Could you check a few things on this model? Use its own coordinates, in mm. Face numbers are marked on the shaded views. Give positions to 0.01 mm unless a question says otherwise; leave off trailing zeros. Loops run counter-clockwise (first coordinate to the right, second up) from the corner with the lowest first, then second, coordinate; pieces in that order, holes last. Notation, with made-up numbers: (23.25, 25.25) -> (71.25, 25.25) arc R22 ccw to (71.25, 50.25) -> close; hole circle Ø3 at (63.25, 20). An arc over 180 degrees is marked (long way). Write each question's results on one line, items separated by ' | '. Start each with the question number.
Q1. If we section it at C-C, the plane y = 322.5: List the corners of the cut face in (x, z) for me, plus the area to 3 significant figures.
Q2. If we section it at B-B, the plane x = 200: List the corners of the cut face in (y, z) for me, plus the area to 3 significant figures.
Q3. If we section it at D-D, the plane y = 122: List the corners of the cut face in (x, z) for me, plus the area to 3 significant figures.
Q4. Will these pins go through, and if not, where does the flat tip stop? P1, Ø12, axis at y = 168, z = 24.5, coming from the -X side; P2, Ø8, axis at x = 69.5, y = 121.5, coming from the +Z side; P3, Ø6.5, axis at y = 346.5, z = 16.5, coming from the -X side; P4, Ø4, axis at y = 351.47, z = 38.1, coming from the +X side.
Q5. If I drill on line 1 along Z through (x, y) = (76.5, 195.5); line 2 along X through (y, z) = (114, 5.5); line 3 along X through (y, z) = (356, 54), over which ranges is the centre line in solid material (lowest first)?
Q6. We'd pull the mould along Y, two halves only. Please class the marked faces 1, 2 and 3: released by +Y, released by -Y, zero draft, split by the parting line, or undercut.
Q7. If we section it at A-A, the plane z = 20: List the corners of the cut face in (x, y) for me (3 decimals), plus the area to 3 significant figures.
from build123d import *

# Parameters (mm, degrees)
F1_DEPTH = 12.7
F2_W     = 25.4
F2_H     = 50.8
F3_DEPTH = 63.5
F4_SIZE  = 20.32
F5_SIZE  = 17.78
F7_DEPTH = 254
F9_DEPTH = 254


with BuildPart() as f1:
    # F0 (on Top) → F1 (new body)
    with BuildSketch(Plane.XY):
        Polygon((50.8, 190.5), (114.3, 190.5), (114.3, 381), (0, 381), (0, 292.1), (50.8, 292.1), align=None)
        Polygon((114.3, 381), (114.3, 190.5), (177.8, 190.5), (177.8, 292.1), (228.6, 292.1), (228.6, 381), align=None)
        Polygon((0, 88.9), (0, 0), (114.3, 0), (114.3, 190.5), (50.8, 190.5), (50.8, 88.9), align=None)
        Polygon((114.3, 190.5), (114.3, 0), (228.6, 0), (228.6, 88.9), (177.8, 88.9), (177.8, 190.5), align=None)
    extrude(amount=F1_DEPTH)

    # F2 (on Top) → F3 (join)
    with BuildSketch(Plane.XY):
        with Locations((139.7, 339.725)):
            Rectangle(F2_W, F2_H)
        with Locations((88.9, 339.725)):
            Rectangle(F2_W, F2_H)
        with Locations((139.7, 41.275)):
            Rectangle(F2_W, F2_H)
        with Locations((88.9, 41.275)):
            Rectangle(F2_W, F2_H)
    extrude(amount=F3_DEPTH)

    # F4
    f4_edges = [f1.edges().sort_by_distance(p)[0] for p in [
        (101.6, 41.275, 63.5),
        (127, 41.275, 63.5),
        (127, 339.725, 63.5),
        (101.6, 339.725, 63.5),
    ]]
    chamfer(f4_edges, length=F4_SIZE)

    # F5
    f5_edges = [f1.edges().sort_by_distance(p)[0] for p in [
        (127, 339.725, 43.18),
        (101.6, 339.725, 43.18),
        (127, 41.275, 43.18),
        (101.6, 41.275, 43.18),
    ]]
    chamfer(f5_edges, length=F5_SIZE)

    # F6 (on face) → F7 (cut)
    with BuildSketch(Plane(origin=(76.2, 0, 0), x_dir=(0, -1, 0), z_dir=(-1, 0, 0))):
        with BuildLine():
            ThreePointArc((-40.005, 48.1965), (-40.3769743879, 49.0945256121), (-41.275, 49.4665))
            Line((-41.275, 49.4665), (-41.275, 46.9265))
            ThreePointArc((-41.275, 46.9265), (-40.3769743879, 47.2984743879), (-40.005, 48.1965))
        make_face()
        with BuildLine():
            Line((-41.275, 46.9265), (-41.275, 49.4665))
            ThreePointArc((-41.275, 49.4665), (-42.545, 48.1965), (-41.275, 46.9265))
        make_face()
        with BuildLine():
            ThreePointArc((-51.7525, 38.1), (-53.0225, 39.37), (-54.2925, 38.1))
            Line((-54.2925, 38.1), (-51.7525, 38.1))
        make_face()
        with BuildLine():
            Line((-51.7525, 38.1), (-54.2925, 38.1))
            ThreePointArc((-54.2925, 38.1), (-53.0225, 36.83), (-51.7525, 38.1))
        make_face()
        with BuildLine():
            ThreePointArc((-39.243, 38.1), (-39.8381590206, 39.5368409794), (-41.275, 40.132))
            Line((-41.275, 40.132), (-41.275, 38.1))
            Line((-41.275, 38.1), (-39.243, 38.1))
        make_face()
        with BuildLine():
            Line((-41.275, 38.1), (-41.275, 40.132))
            ThreePointArc((-41.275, 40.132), (-42.7118409794, 39.5368409794), (-43.307, 38.1))
            Line((-43.307, 38.1), (-41.275, 38.1))
        make_face()
        with BuildLine():
            Line((-41.275, 38.1), (-43.307, 38.1))
            ThreePointArc((-43.307, 38.1), (-42.7118409794, 36.6631590206), (-41.275, 36.068))
            Line((-41.275, 36.068), (-41.275, 38.1))
        make_face()
        with BuildLine():
            ThreePointArc((-41.275, 29.2735), (-42.545, 28.0035), (-41.275, 26.7335))
            Line((-41.275, 26.7335), (-41.275, 29.2735))
        make_face()
        with BuildLine():
            Line((-41.275, 29.2735), (-41.275, 26.7335))
            ThreePointArc((-41.275, 26.7335), (-40.3769743879, 27.1054743879), (-40.005, 28.0035))
            ThreePointArc((-40.005, 28.0035), (-40.3769743879, 28.9015256121), (-41.275, 29.2735))
        make_face()
        with BuildLine():
            Line((-30.7975, 38.1), (-28.2575, 38.1))
            ThreePointArc((-28.2575, 38.1), (-29.5275, 39.37), (-30.7975, 38.1))
        make_face()
        with BuildLine():
            ThreePointArc((-30.7975, 38.1), (-29.5275, 36.83), (-28.2575, 38.1))
            Line((-28.2575, 38.1), (-30.7975, 38.1))
        make_face()
        with BuildLine():
            ThreePointArc((-41.275, 36.068), (-39.8381590206, 36.6631590206), (-39.243, 38.1))
            Line((-39.243, 38.1), (-41.275, 38.1))
            Line((-41.275, 38.1), (-41.275, 36.068))
        make_face()
    extrude(amount=-F7_DEPTH, mode=Mode.SUBTRACT)

    # F8 (on face) → F9 (cut)
    with BuildSketch(Plane(origin=(76.2, 0, 0), x_dir=(0, -1, 0), z_dir=(-1, 0, 0))):
        with BuildLine():
            ThreePointArc((-338.455, 48.1965), (-338.8269743879, 49.0945256121), (-339.725, 49.4665))
            Line((-339.725, 49.4665), (-339.725, 46.9265))
            ThreePointArc((-339.725, 46.9265), (-338.8269743879, 47.2984743879), (-338.455, 48.1965))
        make_face()
        with BuildLine():
            Line((-339.725, 46.9265), (-339.725, 49.4665))
            ThreePointArc((-339.725, 49.4665), (-340.995, 48.1965), (-339.725, 46.9265))
        make_face()
        with BuildLine():
            Line((-350.2025, 38.1), (-352.7425, 38.1))
            ThreePointArc((-352.7425, 38.1), (-351.4725, 36.83), (-350.2025, 38.1))
        make_face()
        with BuildLine():
            ThreePointArc((-350.2025, 38.1), (-351.4725, 39.37), (-352.7425, 38.1))
            Line((-352.7425, 38.1), (-350.2025, 38.1))
        make_face()
        with BuildLine():
            Line((-339.725, 38.1), (-339.725, 40.132))
            ThreePointArc((-339.725, 40.132), (-341.1618409794, 39.5368409794), (-341.757, 38.1))
            Line((-341.757, 38.1), (-339.725, 38.1))
        make_face()
        with BuildLine():
            ThreePointArc((-339.725, 36.068), (-338.2881590206, 36.6631590206), (-337.693, 38.1))
            Line((-337.693, 38.1), (-339.725, 38.1))
            Line((-339.725, 38.1), (-339.725, 36.068))
        make_face()
        with BuildLine():
            ThreePointArc((-337.693, 38.1), (-338.2881590206, 39.5368409794), (-339.725, 40.132))
            Line((-339.725, 40.132), (-339.725, 38.1))
            Line((-339.725, 38.1), (-337.693, 38.1))
        make_face()
        with BuildLine():
            Line((-339.725, 38.1), (-341.757, 38.1))
            ThreePointArc((-341.757, 38.1), (-341.1618409794, 36.6631590206), (-339.725, 36.068))
            Line((-339.725, 36.068), (-339.725, 38.1))
        make_face()
        with BuildLine():
            Line((-329.2475, 38.1), (-326.7075, 38.1))
            ThreePointArc((-326.7075, 38.1), (-327.9775, 39.37), (-329.2475, 38.1))
        make_face()
        with BuildLine():
            ThreePointArc((-329.2475, 38.1), (-327.9775, 36.83), (-326.7075, 38.1))
            Line((-326.7075, 38.1), (-329.2475, 38.1))
        make_face()
        with BuildLine():
            Line((-339.725, 29.2735), (-339.725, 26.7335))
            ThreePointArc((-339.725, 26.7335), (-338.8269743879, 27.1054743879), (-338.455, 28.0035))
            ThreePointArc((-338.455, 28.0035), (-338.8269743879, 28.9015256121), (-339.725, 29.2735))
        make_face()
        with BuildLine():
            ThreePointArc((-339.725, 29.2735), (-340.995, 28.0035), (-339.725, 26.7335))
            Line((-339.725, 26.7335), (-339.725, 29.2735))
        make_face()
    extrude(amount=-F9_DEPTH, mode=Mode.SUBTRACT)


solid = f1.part
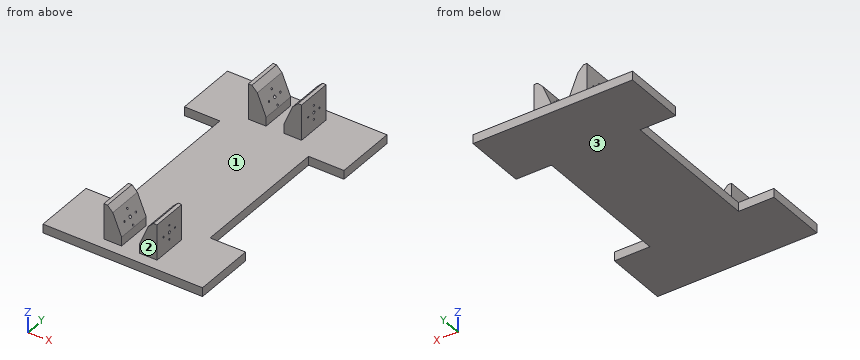
Final values:
1) outline: (0, 0) -> (228.6, 0) -> (228.6, 12.7) -> (152.4, 12.7) -> (152.4, 63.5) -> (147.32, 63.5) -> (139.57, 55.75) -> (127, 25.4) -> (127, 12.7) -> (101.6, 12.7) -> (101.6, 25.4) -> (89.03, 55.75) -> (81.28, 63.5) -> (76.2, 63.5) -> (76.2, 12.7) -> (0, 12.7) -> close | area: 4,850 mm²
2) outline: (0, 0) -> (88.9, 0) -> (88.9, 12.7) -> (0, 12.7) -> close; (292.1, 0) -> (381, 0) -> (381, 12.7) -> (292.1, 12.7) -> close | area: 2,260 mm²
3) outline: (50.8, 0) -> (177.8, 0) -> (177.8, 12.7) -> (50.8, 12.7) -> close | area: 1,610 mm²
4) P1: passes through | P2: stops at z = 12.7 | P3: stops at x = 76.2 | P4: stops at x = 152.4
5) line 1: z = 0 to 12.7 | line 2: x = 50.8 to 177.8 | line 3: x = 76.2 to 89.75, 138.85 to 152.4
6) face 1: undercut | face 2: released by -Y | face 3: zero draft
7) outline: (76.2, 15.875) -> (101.6, 15.875) -> (101.6, 66.675) -> (76.2, 66.675) -> close; (76.2, 314.325) -> (101.6, 314.325) -> (101.6, 365.125) -> (76.2, 365.125) -> close; (127, 15.875) -> (152.4, 15.875) -> (152.4, 66.675) -> (127, 66.675) -> close; (127, 314.325) -> (152.4, 314.325) -> (152.4, 365.125) -> (127, 365.125) -> close | area: 5,160 mm²
